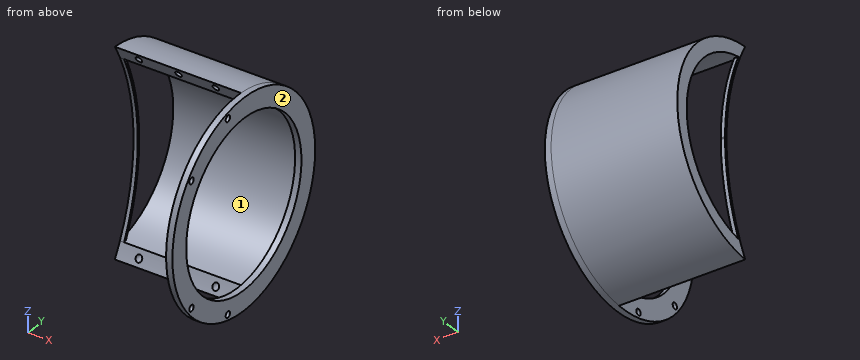
```python
from build123d import *
from build123d.topology import SkipClean

# Parameters (mm, degrees)
SKETCH_1_R      = 49.171750004
SKETCH_1_R_2    = 39.7
EXTRUDE_1_DEPTH = 3
EXTRUDE_START   = 60
EXTRUDE_2_DEPTH = 60
SKETCH_3_R      = 1.5
EXTRUDE_4_DEPTH = 60
EXTRUDE_5_DEPTH = 2
SKETCH_5_R      = 1.5
EXTRUDE_6_DEPTH = 10


with BuildPart() as part:
    # Эскиз1 → Выдавливание1 (new body)
    with BuildSketch(Plane.YZ):
        with Locations(Location((37.5, 47.7, 0), (0, 0, 90))):
            Circle(SKETCH_1_R)
        with Locations(Location((37.5, 47.7, 0), (0, 0, 90))):
            Circle(SKETCH_1_R_2, mode=Mode.SUBTRACT)
    extrude(amount=EXTRUDE_1_DEPTH)

    # Эскиз2 → Выдавливание2 (add)
    with BuildSketch(Plane(origin=(0, 37.5, 47.7), x_dir=(0, 0, 1), z_dir=(-1, 0, 0)).offset(EXTRUDE_START)):
        with BuildLine():
            ThreePointArc((-42.287817796, 5.918654073), (-45.733949258, 4.2292184), (-49.112714544, 2.408789856))
            ThreePointArc((-49.112714544, 2.408789856), (0, 49.171750004), (49.112714544, 2.408789856))
            ThreePointArc((49.112714544, 2.408789856), (45.733949258, 4.2292184), (42.287817796, 5.918654073))
            ThreePointArc((42.287817796, 5.918654073), (0, 42.7), (-42.287817796, 5.918654073))
        make_face()
    extrude(amount=-EXTRUDE_2_DEPTH)

    # Эскиз3 → Выдавливание4 (cut)
    with BuildSketch(Plane(origin=(3, 37.5, 47.7), x_dir=(0, 0, -1), z_dir=(1, 0, 0))):
        with Locations((45.186031447, -10.975999366)):
            Circle(SKETCH_3_R)
        with Locations((29.39321752, -36.031774364)):
            Circle(SKETCH_3_R)
        with Locations((-29.39321752, -36.031774364)):
            Circle(SKETCH_3_R)
        with Locations((-45.186031447, -10.975999366)):
            Circle(SKETCH_3_R)
    extrude(amount=-EXTRUDE_4_DEPTH, mode=Mode.SUBTRACT)

    # Эскиз4 → Выдавливание5 (add)
    with SkipClean():  # the faces are left unmerged after this step: merging them gives an invalid solid
        with BuildSketch(Plane(origin=(-60, 37.5, 47.7), x_dir=(0, 0, 1), z_dir=(-1, 0, 0))):
            with BuildLine():
                Line((-0.24997743, 16.30888643), (0.499998469, 16.307958241))
                Line((0.499998469, 16.307958241), (0, 16.309195752))
                ThreePointArc((0, 16.309195752), (-0.124988811, 16.309118421), (-0.24997743, 16.30888643))
            make_face()
            with BuildLine():
                ThreePointArc((-42.287817796, 5.918654073), (0, 15.3), (42.287817796, 5.918654073))
                Line((42.287817796, 5.918654073), (42.121404236, 7.107651815))
                ThreePointArc((42.121404236, 7.107651815), (21.801545856, 13.928343922), (0.499998469, 16.307958241))
                Line((0.499998469, 16.307958241), (-0.24997743, 16.30888643))
                ThreePointArc((-0.24997743, 16.30888643), (-21.679464377, 13.955250498), (-42.121404236, 7.107651815))
                Line((-42.121404236, 7.107651815), (-42.287817796, 5.918654073))
            make_face()
            with BuildLine():
                Line((0, 16.309195752), (0.499998469, 16.307958241))
                ThreePointArc((0.499998469, 16.307958241), (0.25, 16.308886374), (0, 16.309195752))
            make_face()
        extrude(amount=-EXTRUDE_5_DEPTH)

    # Эскиз5 → Резьба6 (cut)
    with SkipClean():  # the faces are left unmerged after this step: merging them gives an invalid solid
        with BuildSketch(Plane(origin=(1.5, 35.097404478, 62.473935176), x_dir=(0, 0, -1), z_dir=(0, 1, 0))):
            with Locations((-31.126064824, 51.234)):
                Circle(SKETCH_5_R)
            with Locations((-31.126064824, 32.434)):
                Circle(SKETCH_5_R)
            with Locations((-31.126064824, 14.694)):
                Circle(SKETCH_5_R)
            with Locations((60.673935176, 51.234)):
                Circle(SKETCH_5_R)
            with Locations((60.673935176, 32.434)):
                Circle(SKETCH_5_R)
            with Locations((60.673935176, 14.694)):
                Circle(SKETCH_5_R)
        extrude(amount=EXTRUDE_6_DEPTH, mode=Mode.SUBTRACT)


solid = part.part
```
Geometry: final body of the model. Coordinates: model frame, mm. Face numbers are marked on the shaded views. Round coordinates to 2 decimals unless told otherwise and drop trailing zeros. Order: outer loops, then holes, each group sorted by start corner. A loop starts at its lowest first (then second) coordinate and runs counter-clockwise, first axis right, second up. Notation, with made-up numbers: M 52,63.5 L 72,63.5 A23 cw 72,96.5 Z; hole C 36,2.25 d6. An arc over 180 degrees is marked long. One line per item, written item: value.
(1) Cut plane A-A (y = 37.5). Return the cut outline in (x, z).
Result sheet:
outline: M 0,-1.47 L 3,-1.47 L 3,8 L 0,8 Z; M 0,87.4 L 3,87.4 L 3,96.87 L 0,96.87 Z
(2) Line query: probe 1 along Z at (x, y) = (-17, 46); probe 2 along Z at (x, y) = (-27.5, 51.5); probe 3 along X at (y, z) = (43, 1). Output: solid intervals per line, ascending. Write a range as [from, to].
Result sheet:
probe 1: [-0.73, 5.85], [89.55, 96.13]
probe 2: [0.56, 7.36], [88.04, 94.84]
probe 3: [-60, -51], [-48.47, -32.2], [-29.67, -14.46], [-11.93, 3]
(3) Cut plane D-D (y = -4.5). Return the cut outline in (x, z).
Result sheet:
outline: M 0,22.13 L 3,22.13 L 3,73.27 L 0,73.27 Z
(4) Cut plane C-C (x = -6). Return the cut outline in (y, z), and give its area (3 significant figures).
Result sheet:
outline: M 39.91,-1.41 A49.17 ccw 39.91,96.81 A100 cw 43.42,89.99 A42.7 cw 43.42,5.41 A100 cw Z
area: 879 mm2
(5) Pull-direction query (Z, two-part tool) for the marked faces 1 and 2; classes: pulls with the +Z half, pulls with the -Z half, needs draft (parallel to the pull), parting line crosses it, or undercut.
Result sheet:
face 1: undercut
face 2: needs draft
(6) Cut plane B-B (z = 68.5). Return the cut outline in (x, y).
Result sheet:
outline: M -60,50.61 L -58,50.61 L -58,51.64 L -60,51.64 Z; M -60,74.79 L 0,74.79 L 0,71.31 L 3,71.31 L 3,82.06 L -60,82.06 Z; M 0,-7.06 L 3,-7.06 L 3,3.69 L 0,3.69 Z
(7) Pin query (flat end, axial travel): P1, Ø2.5, axis at y = 1.47, z = 18.31, coming from the +X side; P2, Ø2.5, axis at x = -13.5, z = 94, coming from the -Y side; P3, Ø1, axis at x = -48, z = 56.5, coming from the -Y side; P4, Ø5, axis at x = -13.194, z = 93.6, coming from the +Y side. Return the tip coordinate at first contact, or that it passes through.
Result sheet:
P1: through
P2: y = 40.77
P3: y = 79.17
P4: y = 60.61
